from build123d import *

# Parameters (mm, degrees)
F0_W     = 7.9375
F0_H     = 7.9375
F0_R     = 2.38125
F1_DEPTH = 9.525
F2_DEPTH = 11.1125
F3_T     = -1.5875


with BuildPart() as f1:
    # F0 (on Top) → F1 (new body)
    with BuildSketch(Plane.XY):
        Rectangle(F0_W, F0_H)
        Circle(F0_R, mode=Mode.SUBTRACT)
    extrude(amount=F1_DEPTH)

    # F0 (on Top) → F2 (join)
    with BuildSketch(Plane.XY):
        Circle(F0_R)
    extrude(amount=F2_DEPTH)

    # F3
    f3_openings = [f1.faces().sort_by_distance(p)[0] for p in [
        (0, 0, 0),
    ]]
    offset(amount=F3_T, openings=f3_openings, kind=Kind.INTERSECTION)


solid = f1.part
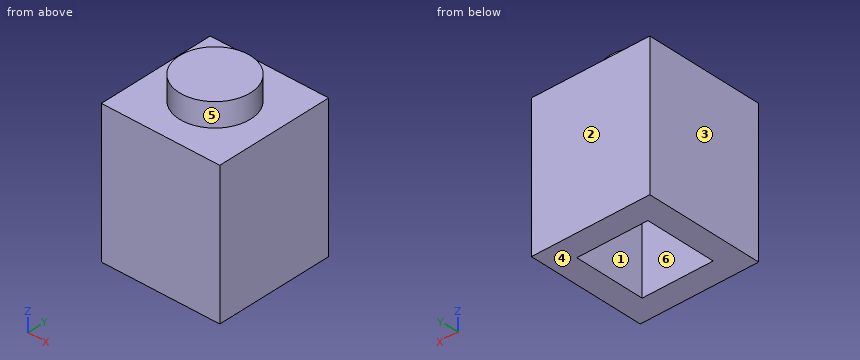
Source: CAD feature listing. Evaluate the final solid. Frame: model axes, mm. Face numbers are marked on the shaded views. A direction names the side the tool comes from. Coordinates: 2 decimals unless noted, no trailing zeros. Loops run counter-clockwise (first coordinate to the right, second up) from the corner with the lowest first, then second, coordinate; pieces in that order, holes last. Notation, with made-up numbers: M 10.5,-16 L 59.5,-16 A16 ccw 59.5,6 Z; hole C 44,27.5 d5. An arc over 180 degrees is marked long. Answer in a Markdown table with one row per item.
Q1. Ray query, probe 1 along X at (y, z) = (1.75, 3); probe 2 along X at (y, z) = (0, 8.6). Return the intervals inside material, ascending. Write a range as from..to.
Answers below:
| item | result |
|---|---|
| probe 1 | x = -3.97..-2.38, 2.38..3.97 |
| probe 2 | x = -3.97..-0.79, 0.79..3.97 |
Q2. Section B-B on y = 0. Return the cut outline in (x, z) (1 decimal).
Answers below:
| item | result |
|---|---|
| outline | M -4,0 L -2.4,0 L -2.4,7.9 L -0.8,7.9 L -0.8,9.5 L 0.8,9.5 L 0.8,7.9 L 2.4,7.9 L 2.4,0 L 4,0 L 4,9.5 L 2.4,9.5 L 2.4,11.1 L -2.4,11.1 L -2.4,9.5 L -4,9.5 Z |
Q3. Draft query along Y for the marked faces 1, 2 and 3. Return one class per face: pulls with the +Y half, pulls with the -Y half, needs draft (parallel to the pull), parting line crosses it, or undercut.
Answers below:
| item | result |
|---|---|
| face 1 | undercut |
| face 2 | pulls with the +Y half |
| face 3 | needs draft |
Q4. Section A-A on z = 1.25. Return the cut outline in (x, y).
Answers below:
| item | result |
|---|---|
| outline | M -3.97,-3.97 L 3.97,-3.97 L 3.97,3.97 L -3.97,3.97 Z; hole M -2.38,-2.38 L 2.38,-2.38 L 2.38,2.38 L -2.38,2.38 Z |
Q5. First-contact query: pin 1 (2.5 mm diameter, centred on x = 1, y = 0, fed in from -Z); pin 2 (0.5 mm diameter, centred on x = 0, y = 0, fed in from -Z) (3 decimals). Flat tips, straight axial feed; report the tip coordinate or a pass-through.
Answers below:
| item | result |
|---|---|
| pin 1 | stops at z = 7.94 |
| pin 2 | stops at z = 9.525 |
Q6. Section D-D on z = 8.25. Return the cut outline in (x, y).
Answers below:
| item | result |
|---|---|
| outline | M -3.97,-3.97 L 3.97,-3.97 L 3.97,3.97 L -3.97,3.97 Z; hole C 0,0 d1.59 |
Q7. Set-up query: the marked faces 4, 5 and 6. Return all of +Z, -Z, +X, -X, +Y, -Y with unobstructed straight access to the full face (end or side cutting, diameter ignored); none if empty.
Answers below:
| item | result |
|---|---|
| face 4 | -Z, +X, -X, +Y, -Y |
| face 5 | +Z |
| face 6 | -Z |
